Can you work these out from the model? Positions are in its coordinate system, mm. A direction names the side the tool comes from. Give positions to 0.01 mm unless a question says otherwise; leave off trailing zeros. Order: outer loops, then holes, each group sorted by start corner. A loop starts at its lowest first (then second) coordinate and runs counter-clockwise, first axis right, second up. Notation, with made-up numbers: (63, 4.25) - (83, 4.25) arc R21 ccw to (83, 27.25) - close; hole circle Ø2 at (26, -11). An arc over 180 degrees is marked (long way). Answer as a JSON object with one key per item and string values.
```python
from build123d import *

# Parameters (mm, degrees)
F1_DEPTH = 100
F2_DEPTH = 75
F3_DEPTH = 25


with BuildPart() as f1:
    # F0 (on Top) → F1 (new body)
    with BuildSketch(Plane.XY):
        Polygon((-107.777781, 0), (-97.777781, 0), (102.222219, 0), (102.222219, 10), (38, 10), (-12.328933, 10), (-68.002172, 10), (-97.777781, 10), (-97.777781, 140), (-107.777781, 140), align=None)
    extrude(amount=F1_DEPTH)

    # F0 (on Top) → F2 (join)
    with BuildSketch(Plane.XY):
        with BuildLine():
            Line((-12.328933, 10), (38, 10))
            ThreePointArc((38, 10), (107.714757, 79.714757), (38, 149.429513))
            Line((38, 149.429513), (0, 149.429513))
            Line((0, 149.429513), (0, 53.262483))
            Line((0, 53.262483), (-60.966311, 149.429513))
            Line((-60.966311, 149.429513), (-97.777781, 140))
            Line((-97.777781, 140), (-97.777781, 10))
            Line((-97.777781, 10), (-68.002172, 10))
            Line((-68.002172, 10), (-68.002172, 35.399918))
            Line((-68.002172, 35.399918), (-33.959807, 44.120105))
            Line((-33.959807, 44.120105), (-12.328933, 10))
        make_face()
        Polygon((-46.412745, 68.920866), (-68.002172, 63.875206), (-68.002172, 102.975592), align=None, mode=Mode.SUBTRACT)
        with BuildLine():
            Line((38, 45.601577), (38, 114.87817))
            ThreePointArc((38, 114.87817), (72.638297, 80.239873), (38, 45.601577))
        make_face(mode=Mode.SUBTRACT)
    extrude(amount=F2_DEPTH)

    # F0 (on Top) → F3 (cut)
    with BuildSketch(Plane.XY):
        with BuildLine():
            Line((-12.328933, 10), (38, 10))
            ThreePointArc((38, 10), (107.714757, 79.714757), (38, 149.429513))
            Line((38, 149.429513), (0, 149.429513))
            Line((0, 149.429513), (0, 53.262483))
            Line((0, 53.262483), (-60.966311, 149.429513))
            Line((-60.966311, 149.429513), (-97.777781, 140))
            Line((-97.777781, 140), (-97.777781, 10))
            Line((-97.777781, 10), (-68.002172, 10))
            Line((-68.002172, 10), (-68.002172, 35.399918))
            Line((-68.002172, 35.399918), (-33.959807, 44.120105))
            Line((-33.959807, 44.120105), (-12.328933, 10))
        make_face()
        Polygon((-46.412745, 68.920866), (-68.002172, 63.875206), (-68.002172, 102.975592), align=None, mode=Mode.SUBTRACT)
        with BuildLine():
            Line((38, 45.601577), (38, 114.87817))
            ThreePointArc((38, 114.87817), (72.638297, 80.239873), (38, 45.601577))
        make_face(mode=Mode.SUBTRACT)
    extrude(amount=F3_DEPTH, mode=Mode.SUBTRACT)


solid = f1.part
```
Q1. If we section it at D-D, the plane y = 20: Please give me the cut outline in (x, z), then the cut area to 3 significant figures.
Recorded:
{"outline": "(-107.78, 0) - (-97.78, 0) - (-97.78, 25) - (-68, 25) - (-68, 75) - (-97.78, 75) - (-97.78, 100) - (-107.78, 100) - close; (-18.67, 25) - (73.98, 25) - (73.98, 75) - (-18.67, 75) - close", "area": "7,120 mm^2"}
Q2. I need wall thicknesses on L1, parallel to X at y = 57.5, z = 51; L2, parallel to X at y = 82.5, z = 30; L3, parallel to X at y = 60.5, z = 56. Which ranges of each line are inside material? Lowest first, please.
Recorded:
{"L1": "x = -107.78 to -2.69, 0 to 38, 64.13 to 104.08", "L2": "x = -107.78 to -68, -55.02 to -18.54, 0 to 38, 72.56 to 107.66", "L3": "x = -107.78 to -4.59, 0 to 38, 66.46 to 105.01"}
Q3. If we section it at A-A, the plane z = 27.5: Please give me the cut outline in (x, y), then the cut area to 3 significant figures.
Recorded:
{"outline": "(-107.78, 0) - (102.22, 0) - (102.22, 10) - (38, 10) arc R69.71 ccw to (38, 149.43) - (0, 149.43) - (0, 53.26) - (-60.97, 149.43) - (-97.78, 140) - (-107.78, 140) - close; hole (-68, 10) - (-12.33, 10) - (-33.96, 44.12) - (-68, 35.4) - close; hole (-68, 63.88) - (-46.41, 68.92) - (-68, 102.98) - close; hole (38, 45.6) arc R34.64 ccw to (38, 114.88) - close", "area": "23,200 mm^2"}
Q4. I'm going to push flat-ended pins straight in: pin 1 Ø6 at (x, y) = (-22.5, 51.5) entering from -Z; pin 2 Ø2 at (y, z) = (117, 75.5) entering from +X; pin 3 Ø20 at (y, z) = (73, 8) entering from +X. Where does each tip first touch, or does it pass through?
Recorded:
{"pin 1": "stops at z = 25", "pin 2": "stops at x = 97.45", "pin 3": "stops at x = -97.78"}
Q5. If we section it at B-B, the plane y = 128: Please give me the cut outline in (x, z), then the cut area to 3 significant figures.
Recorded:
{"outline": "(-107.78, 0) - (-97.78, 0) - (-97.78, 25) - (-47.38, 25) - (-47.38, 75) - (-97.78, 75) - (-97.78, 100) - (-107.78, 100) - close; (0, 25) - (88.29, 25) - (88.29, 75) - (0, 75) - close", "area": "7,930 mm^2"}
Q6. Which directions (+Z, -Z, +X, -X, +Y, -Y) give clear straight access to the entire face, cutting with the end or side of a thin tool? Please do faces 5 (the face through (72.63, 81, 49.65)), 6 (the face through (102.222, 5, 49)), 7 (the face through (0, 102, 50)), 8 (the face through (-103, 140, 49)).
Recorded:
{"face 5": "+Z, -Z", "face 6": "+Z, -Z, +X, -Y", "face 7": "+Z, -Z, +Y", "face 8": "+Z, -Z, -X, +Y"}
Q7. We'd pull the mould along Y, two halves only. Please class faces 1 (the face through (-97.778, 74, 87)), 2 (the face through (-30.056, 100.673, 49.65)), 3 (the face through (-57.36, 86.19, 49.65)), 4 (the face through (107.7, 78.2, 49.6)): released by +Y, released by -Y, zero draft, split by the parting line, or undercut.
Recorded:
{"face 1": "zero draft", "face 2": "released by +Y", "face 3": "undercut", "face 4": "undercut"}
Q8. If we section it at C-C, the plane x = 25: Please give me the cut outline in (y, z).
Recorded:
{"outline": "(0, 0) - (10, 0) - (10, 25) - (149.43, 25) - (149.43, 75) - (10, 75) - (10, 100) - (0, 100) - close"}
